```python
from build123d import *

# Parameters (mm, degrees)
SKETCH_1_W          = 48
SKETCH_1_H          = 20
EXTRUDE_1_DEPTH     = 30
SKETCH_2_W          = 14
SKETCH_2_H          = 30
CUT_EXTRUDE_1_DEPTH = 7
SKETCH_7_W          = 22
SKETCH_7_H          = 30
EXTRUDE_2_DEPTH     = 48
SKETCH_8_W          = 21
SKETCH_8_H          = 30
CUT_EXTRUDE_2_DEPTH = 14
SKETCH_9_W          = 21
SKETCH_9_H          = 30
CUT_EXTRUDE_3_DEPTH = 14
SKETCH_11_W         = 10.2
SKETCH_11_H         = 20.2
CUT_EXTRUDE_4_DEPTH = 56.497747702
SKETCH_13_R         = 4.1
CUT_EXTRUDE_5_DEPTH = 44.783558558
FILLET_1_R          = 7
SKETCH1_W           = 10.2
SKETCH1_H           = 20.2
BOSS_EXTRUDE1_DEPTH = 4
SKETCH2_W           = 20
SKETCH2_H           = 21
CUT_EXTRUDE1_DEPTH  = 51
SKETCH3_R           = 11.3
CUT_EXTRUDE2_DEPTH  = 40.962482405


with BuildPart() as part:
    # Эскиз1 → Бобышка-Вытянуть1 (new body)
    with BuildSketch(Plane(origin=(0, 0, 0), x_dir=(1, 0, 0), z_dir=(0, 1, 0))):
        Rectangle(SKETCH_1_W, SKETCH_1_H)
    extrude(amount=EXTRUDE_1_DEPTH)

    # Эскиз2 → Вырез-Вытянуть1 (cut)
    with BuildSketch(Plane.XY.offset(10)):
        with Locations((0, 15)):
            Rectangle(SKETCH_2_W, SKETCH_2_H)
    extrude(amount=-CUT_EXTRUDE_1_DEPTH, mode=Mode.SUBTRACT)

    # Эскиз7 → Бобышка-Вытянуть2 (add)
    with BuildSketch(Plane(origin=(24, 0, 0), x_dir=(0, 0, -1), z_dir=(1, 0, 0))):
        with Locations((21, 15)):
            Rectangle(SKETCH_7_W, SKETCH_7_H)
    extrude(amount=-EXTRUDE_2_DEPTH)

    # Эскиз8 → Вырез-Вытянуть2 (cut)
    with BuildSketch(Plane(origin=(24, 0, 0), x_dir=(0, 0, -1), z_dir=(1, 0, 0))):
        with Locations((21.5, 15)):
            Rectangle(SKETCH_8_W, SKETCH_8_H)
    extrude(amount=-CUT_EXTRUDE_2_DEPTH, mode=Mode.SUBTRACT)

    # Эскиз9 → Вырез-Вытянуть3 (cut)
    with BuildSketch(Plane.ZY.offset(24)):
        with Locations((-21.5, 15)):
            Rectangle(SKETCH_9_W, SKETCH_9_H)
    extrude(amount=-CUT_EXTRUDE_3_DEPTH, mode=Mode.SUBTRACT)

    # Эскиз11 → Вырез-Вытянуть4 (cut, through all)
    with BuildSketch(Plane.ZY.offset(10)):
        with Locations((-21.5, 15)):
            Rectangle(SKETCH_11_W, SKETCH_11_H)
    extrude(amount=-CUT_EXTRUDE_4_DEPTH, mode=Mode.SUBTRACT)

    # Эскиз13 → Вырез-Вытянуть5 (cut, through all)
    with BuildSketch(Plane(origin=(0, 0, -11), x_dir=(-1, 0, 0), z_dir=(0, 0, -1))):
        with Locations((17, 15)):
            Circle(SKETCH_13_R)
        with Locations((-17, 15)):
            Circle(SKETCH_13_R)
    extrude(amount=-CUT_EXTRUDE_5_DEPTH, mode=Mode.SUBTRACT)

    # Скругление1
    fillet_1_edges = [part.edges().sort_by_distance(p)[0] for p in [
        (-7, 15, 3),
        (7, 15, 3),
    ]]
    fillet(fillet_1_edges, radius=FILLET_1_R - 0.0001)  # a hair under: the kernel refuses the full size

    # Sketch1 → Boss-Extrude1 (add)
    with BuildSketch(Plane(origin=(10, 0, 0), x_dir=(0, 0, -1), z_dir=(1, 0, 0))):
        with Locations((21.5, 15)):
            Rectangle(SKETCH1_W, SKETCH1_H)
    extrude(amount=-BOSS_EXTRUDE1_DEPTH)

    # Sketch2 → Cut-Extrude1 (cut, through all)
    with BuildSketch(Plane(origin=(0, 30, 0), x_dir=(1, 0, 0), z_dir=(0, 1, 0))):
        with Locations((0, 21.5)):
            Rectangle(SKETCH2_W, SKETCH2_H)
    extrude(amount=-CUT_EXTRUDE1_DEPTH, mode=Mode.SUBTRACT)

    # Sketch3 → Cut-Extrude2 (cut, through all)
    with BuildSketch(Plane(origin=(0, 30, 0), x_dir=(1, 0, 0), z_dir=(0, 1, 0))):
        with Locations((0, -10)):
            Circle(SKETCH3_R)
    extrude(amount=-CUT_EXTRUDE2_DEPTH, mode=Mode.SUBTRACT)


solid = part.part
```
The model under review builds one solid part; all positions refer to its coordinate system, in mm. Coordinates: 2 decimals unless noted, no trailing zeros. Write each loop counter-clockwise with the first axis right and the second up, starting at its lowest first coordinate (ties: lowest second). Pieces come first, ordered by that corner, then holes. Notation, with made-up numbers: (23, -35.75) - (28, -35.75) arc R30 cw to (28, -4.75) - close; hole circle Ø1 at (82.25, -25). An arc over 180 degrees is marked (long way). Write item = value, one per line.
(1) Consider section A-A, the plane y = 15. Give the boundary of the cut face in (x, z).
Result sheet:
outline = (-24, -11) - (-21.1, -11) - (-21.1, 10) - (-24, 10) - close; (-12.9, -11) - (12.9, -11) - (12.9, 10) - (11.3, 10) arc R11.3 cw to (-11.3, 10) - (-12.9, 10) - close; (21.1, -11) - (24, -11) - (24, 10) - (21.1, 10) - close
(2) Mouldability with a two-part tool opening along X and no side actions: class faces 1 (the face through (-19, 11, 10)), 2 (the face through (-12.904, 15.18, -0.647)), 3 (the face through (24, 15, 0)), 4 (the face through (-24, 15, 0)) as pulls with the +X half, pulls with the -X half, needs draft (parallel to the pull), parting line crosses it, or undercut.
Result sheet:
face_1 = needs draft
face_2 = undercut
face_3 = pulls with the +X half
face_4 = pulls with the -X half
(3) For line 1 (Y direction, x = -17, z = -8.5); line 2 (X direction, y = 17, z = 4.75); line 3 (X direction, y = 15.5, z = -4), list the stretches that pass through material, from the lowest coordinate up. Write a range as [from, to].
Result sheet:
line_1 = [0, 10.9], [19.1, 30]
line_2 = [-24, -20.58], [-13.42, -10.01], [10.01, 13.42], [20.58, 24]
line_3 = [-24, -21.07], [-12.93, 12.93], [21.07, 24]
(4) Consider section D-D, the plane z = -9.25. Give the boundary of the cut face in (x, y).
Result sheet:
outline = (-24, 0) - (24, 0) - (24, 30) - (-24, 30) - close; hole circle Ø8.2 at (-17, 15); hole circle Ø8.2 at (17, 15)
(5) Consider section C-C, the plane z = 5.25. Give the boundary of the cut face in (x, y).
Result sheet:
outline = (-24, 0) - (-10.25, 0) - (-10.25, 30) - (-24, 30) - close; (10.25, 0) - (24, 0) - (24, 30) - (10.25, 30) - close; hole circle Ø8.2 at (-17, 15); hole circle Ø8.2 at (17, 15)
(6) Consider section B-B, the plane x = 17. Give the boundary of the cut face in (y, z).
Result sheet:
outline = (0, -11) - (10.9, -11) - (10.9, 10) - (0, 10) - close; (19.1, -11) - (30, -11) - (30, 10) - (19.1, 10) - close
(7) For P1, Ø3, axis at x = 3, y = 16, coming from the +Z side, flat-tipped, find the tip position at first contact; note if it passes through.
Result sheet:
P1 = -0.37
